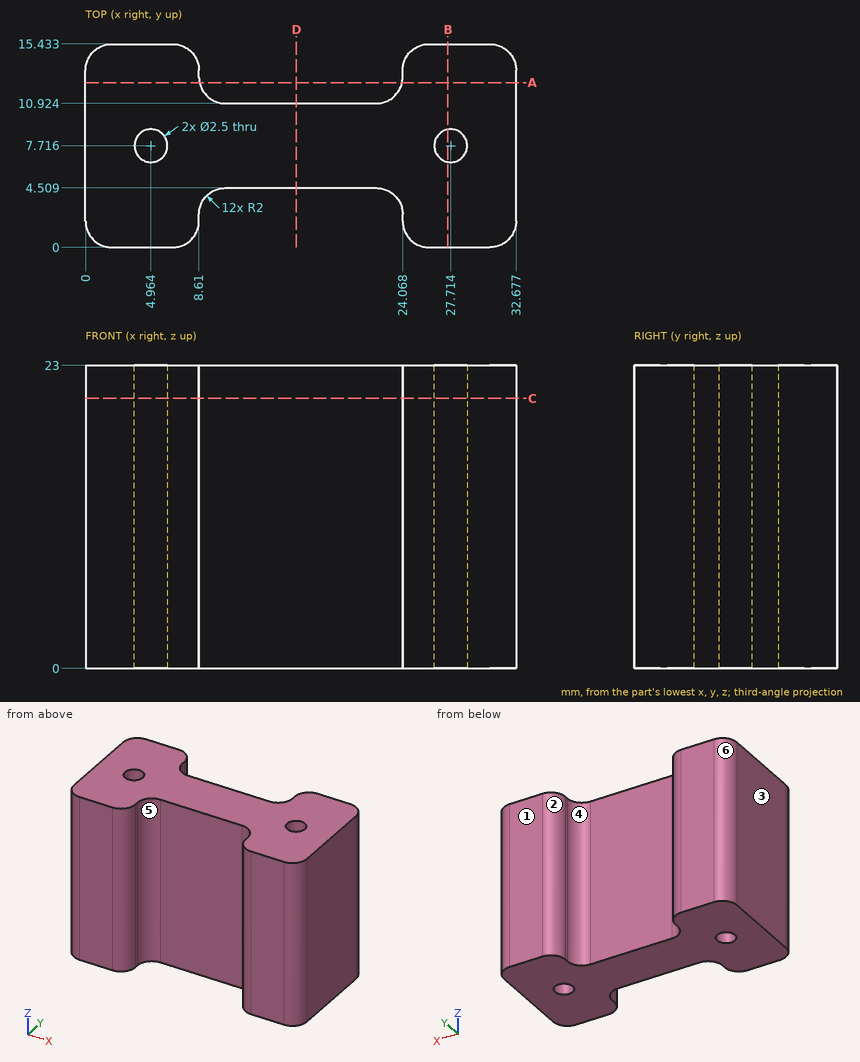
Geometry: see drawing. Coordinates: mm, zero at the bounding-box minimum. A direction names the side the tool comes from. Round coordinates to 2 decimals unless told otherwise and drop trailing zeros. Loops run counter-clockwise (first coordinate to the right, second up) from the corner with the lowest first, then second, coordinate; pieces in that order, holes last. Notation, with made-up numbers: (64.25, -29.5) -> (102.25, -29.5) arc R19 ccw to (102.25, -4.5) -> close; hole circle Ø6 at (-1.5, 87.25). An arc over 180 degrees is marked (long way). One line per question, with ' | ' between items. Start each with the question number.
1. Section B-B on x = 27.5. Output: boundary loops of the cut face in (y, z) (1 decimal).
2. Line query: line 1 along X through (y, z) = (2, 7.25); line 2 along Y through (x, z) = (5, 20.25) (1 decimal); line 3 along X through (y, z) = (8.25, 13.25) (1 decimal). Output: solid intervals per line, ascending. Write a range as [from, to].
3. Section A-A on y = 12.5. Output: boundary loops of the cut face in (x, z) (1 decimal).
4. Mould query, pull axis X, two halves, no side actions, for the marked faces 1, 2 and 3. Classes: pulls with the +X half, pulls with the -X half, needs draft (parallel to the pull), parting line crosses it, or undercut.
5. Set-up query: the marked faces 4, 5 and 6. Return all of +Z, -Z, +X, -X, +Y, -Y with unobstructed straight access to the full face (end or side cutting, diameter ignored); none if empty.
6. Contact query for flat-ended pins moving along their axis: pin 1 (5.5 mm diameter, centred on x = 17, z = 15, fed in from -Y); pin 2 (12.5 mm diameter, centred on x = 15.5, z = 7, fed in from +Y). Output: stop coordinate, or through.
7. Section D-D on x = 16. Output: boundary loops of the cut face in (y, z) (1 decimal).
8. Section C-C on z = 20.5. Count the separate pieces of the cut face and the enclosed holes in it, and give its area (3 significant figures).
Returned:
1) outline: (0, 0) -> (6.5, 0) -> (6.5, 23) -> (0, 23) -> close; (8.9, 0) -> (15.4, 0) -> (15.4, 23) -> (8.9, 23) -> close
2) line 1: x = [0, 8.61], [24.07, 32.68] | line 2: y = [0, 6.5], [9, 15.4] | line 3: x = [0, 3.8], [6.1, 26.6], [28.8, 32.7]
3) outline: (0, 0) -> (8.7, 0) -> (8.7, 23) -> (0, 23) -> close; (24, 0) -> (32.7, 0) -> (32.7, 23) -> (24, 23) -> close
4) face 1: needs draft | face 2: undercut | face 3: pulls with the -X half
5) face 4: +Z, -Z, +Y | face 5: +Z, -Z, -Y | face 6: +Z, -Z, -X, +Y
6) pin 1: stops at y = 4.51 | pin 2: stops at y = 11.46
7) outline: (4.5, 0) -> (10.9, 0) -> (10.9, 23) -> (4.5, 23) -> close
8) separate pieces: 1 | enclosed holes: 2 | area: 352 mm2
